Input: part model. Units: mm. Frame: model coordinates. Face numbers are marked on the shaded views. Give positions to 0.01 mm unless a question says otherwise; leave off trailing zeros. Write each loop counter-clockwise with the first axis right and the second up, starting at its lowest first coordinate (ties: lowest second). Pieces come first, ordered by that corner, then holes.
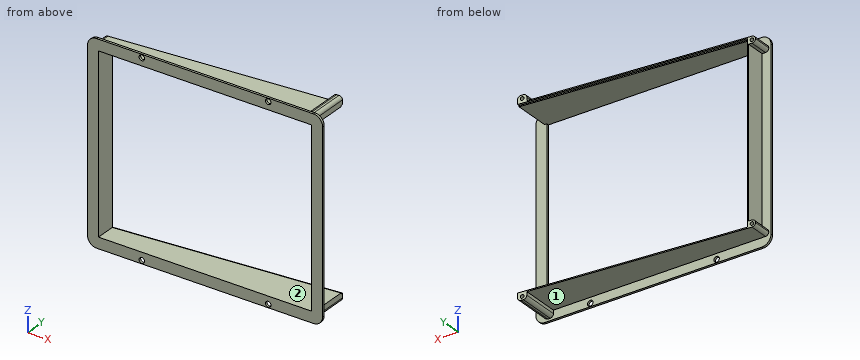
Autodesk Inventor part; units mm, degrees
ref_plane "YZ Plane" through (0, 0, 0) normal (1, 0, 0) x (0, 1, 0)
ref_plane "XZ Plane" through (0, 0, 0) normal (0, 1, 0) x (-1, 0, 0)
ref_plane "XY Plane" through (0, 0, 0) normal (0, 0, 1) x (1, 0, 0)
sketch "panelconnect" plane through (0, 0, 0) normal (0, 1, 0) x (-1, 0, 0)
  circle A0 centre (0, 0) radius 2.5
  circle A1 centre (115, 0) radius 2.5
  circle A2 centre (115, 173) radius 2.5
  circle A3 centre (0, 173) radius 2.5
  line L0 (57.2025, 240.8064) -> (94.1768, 240.8064)
  line L1 (94.1768, 240.8064) -> (82.9725, 250.4701)
  line L2 (82.9725, 250.4701) -> (82.9725, 230.5824)
  line L3 (82.9725, 230.5824) -> (94.1768, 240.8064)
  line L4 (172.5, 184) -> (-57.5, 184)
  line L5 (-57.5, 184) -> (-57.5, -11)
  line L6 (-57.5, -11) -> (172.5, -11)
  line L7 (172.5, -11) -> (172.5, 184)
  line L8 (-39.5, 166) -> (154.5, 166)
  line L9 (154.5, 166) -> (154.5, 7)
  line L10 (154.5, 7) -> (-39.5, 7)
  line L11 (-39.5, 7) -> (-39.5, 166)
  line L12 (164.5, 176) -> (-49.5, 176)
  line L13 (-49.5, 176) -> (-49.5, -3)
  line L14 (-49.5, -3) -> (164.5, -3)
  line L15 (164.5, -3) -> (164.5, 176)
  dimension "d0" = 5
  dimension "d1" = 5
  dimension "d3" = 5
  dimension "d7" = 5
  dimension "d11" = 195
  dimension "d14" = 18
  dimension "d15" = 10
  dimension "d54" = 115
  dimension "d55" = 57.5
  dimension "d56" = 57.5
  dimension "d57" = 230
  dimension "d58" = 173
  dimension "d61" = 11
  dimension "d62" = 57.5
  dimension "d64" = 57.5
  dimension "d65" = 11
extrude "panelExtrude" add sketch "panelconnect" along normal blind 2 contours L15 L14 L13 L12
sketch "Sketch2" plane through (0, 2, 0) normal (0, 1, 0) x (1, 0, 0)
  line L0 (39.5, -7) -> (39.5, -166)
  line L1 (-154.5, -166) -> (39.5, -166)
  line L2 (39.5, -166) -> (39.5, -7)
  line L3 (39.5, -7) -> (-154.5, -7)
  line L4 (-154.5, -7) -> (-154.5, -166)
  line L5 (41.5, -168) -> (-156.5, -168)
  line L6 (-156.5, -168) -> (-156.5, -5)
  line L7 (-156.5, -5) -> (41.5, -5)
  line L8 (41.5, -5) -> (41.5, -168)
  line L9 (39.5, -7) -> (64.2045, -7)
  line L10 (39.5, -166) -> (-154.5, -166)
  line L11 (39.5, -166) -> (69.5542, -166)
  line L12 (-156.5, -5) -> (-156.5, -168)
  line L13 (41.5, -168) -> (33.5, -168)
  line L14 (33.5, -168) -> (33.5, -174)
  line L15 (33.5, -174) -> (41.5, -174)
  line L16 (41.5, -174) -> (41.5, -168)
  line L17 (41.5, -5) -> (33.5, -5)
  line L18 (33.5, -5) -> (33.5, 1)
  line L19 (33.5, 1) -> (41.5, 1)
  line L20 (41.5, 1) -> (41.5, -5)
  circle A0 centre (37.5, -171) radius 1.55
  circle A1 centre (37.5, -2) radius 1.55
  line L21 (-156.5, -168) -> (-162.5, -168)
  line L22 (-162.5, -168) -> (-162.5, -162)
  line L23 (-162.5, -162) -> (-156.5, -162)
  line L24 (-156.5, -162) -> (-156.5, -168)
  line L25 (-156.5, -5) -> (-162.5, -5)
  line L26 (-162.5, -5) -> (-162.5, -11)
  line L27 (-162.5, -11) -> (-156.5, -11)
  line L28 (-156.5, -11) -> (-156.5, -5)
  circle A2 centre (-159.5, -165) radius 1.55
  circle A3 centre (-159.5, -8) radius 1.55
  point P0 (0, 0)
  point P1 (41.5, -166)
  point P2 (41.5, -7)
  point P3 (-156.5, -5)
  dimension "d18" = 2
  dimension "d28" = 8
  dimension "d29" = 6
  dimension "d30" = 6
  dimension "d34" = 3.1
  dimension "d35" = 3
  dimension "d36" = 4
  dimension "d37" = 3.1
  dimension "d38" = 3
  dimension "d39" = 4
  dimension "d42" = 6
  dimension "d43" = 6
  dimension "d44" = 6
  dimension "d45" = 6
  dimension "d46" = 3.1
  dimension "d47" = 3
  dimension "d48" = 3
  dimension "d49" = 3.1
  dimension "d50" = 3
  dimension "d51" = 3
extrude "bodyExtrude" add sketch "Sketch2" along normal blind 35 contours L3 L4 L1 L11 L8 L5 L6 L7 L9 | L7 L18 L19 L20 | L16 L15 L14 L5 | L6 L27 L26 L25 | L21 L22 L23 L6
sketch "Sketch3" plane through (-161.5, 2, 168) normal (0, 0, 1) x (1, 0, 0)
  line L0 (203, 0) -> (203, 35)
  line L1 (203, 35) -> (-34.1829, 14.2492)
  line L2 (203, 35) -> (441.0889, 35) construction
  line L3 (7, 35) -> (203, 35)
  line L4 (-1, 0) -> (-1, 35)
  line L5 (-1, 17.5) -> (-1, 35)
  line L6 (203, 35) -> (195, 35)
  line L7 (-1, 35) -> (203, 35)
  point P0 (161.5, -2)
  point P1 (-1, 17.1523)
  dimension "d22" = 175
extrude "baseAngle" cut sketch "Sketch3" against normal mid plane 398.4625
sketch "Sketch4" plane through (-161.5, 19.2398, 168) normal (-0.0872, 0.9962, 0) x (0.9962, 0.0872, 0)
  line L0 (7.0267, 161) -> (7.0267, 2)
  line L1 (7.0267, 2) -> (203.6093, 2)
  line L2 (203.6093, 2) -> (203.6093, 161)
  line L3 (203.6093, 161) -> (7.0267, 161)
  line L4 (7.0267, 161) -> (7.0267, 2)
  line L5 (6.0267, 162) -> (204.6093, 162)
  line L6 (204.6093, 162) -> (204.6093, 1)
  line L7 (204.6093, 1) -> (6.0267, 1)
  line L8 (6.0267, 1) -> (6.0267, 162)
  point P0 (159.2086, 168)
  point P1 (7.0267, 21.4312)
  dimension "d25" = 1
extrude "bodyDetent" cut sketch "Sketch4" against normal blind 2 contours L3 L2 L1 L0 | L5 L6 L7 L8
fillet "Fillet1" radius 8.35 4 edges at (49.5, 1, -3) (-164.5, 1, -3) (-164.5, 1, 176) (49.5, 1, 176)
fillet "Fillet2" radius 3 8 edges at (33.5, 19.15, 174) (41.5, 19.5, 174) (41.5, 19.5, -1) (33.5, 19.15, -1) (-162.5, 10.5762, 11) (-162.5, 10.5762, 5) (-162.5, 10.5762, 162) (-162.5, 10.5762, 168)
properties part number "mainBody"
Item 1: Section D-D (x = 0). Return loops of the section in (y, z), and give its area (3 significant figures).
Item 2: Section A-A (y = 8). Give the number of separate pieces and of enclosed holes in the cut face, and give its area (3 significant figures).
Item 3: Ray query, line 1 (Z direction, x = 37.5, y = 15); line 2 (Z direction, x = -43, y = 15); line 3 (Z direction, x = -115, y = 0.7). Return the intervals inside material, ascending.
Item 4: Mould query, pull axis Z, two halves, no side actions, for the marked faces 1 and 2. Classes: +Z half, -Z half, draft (parallel to the pull), parting line (faces both ways), or undercut.
Item 5: Section C-C (y = 28.5). Return loops of the section in (x, z).
Item 6: Pin query (flat end, axial travel): pin 1 (1.5 mm diameter, centred on x = 19, y = 33, fed in from -Z); pin 2 (8 mm diameter, centred on x = 0, z = 173, fed in from +Y); pin 3 (9.5 mm diameter, centred on x = -78.5, y = 27, fed in from +Z); pin 4 (4 mm diameter, centred on x = -93, y = 29, fed in from -Z). Return the tip coordinate at first contact, or that it passes through.
Item 7: Section B-B (z = 151). Return loops of the section in (x, y), and give its area (3 significant figures).
Solved:
1. outline: (0, -3) - (2, -3) - (2, -2.5) - (0, -2.5) - close; (0, 2.5) - (2, 2.5) - (2, 5) - (33.37, 5) - (33.37, 6) - (31.36, 6) - (31.36, 7) - (0, 7) - close; (0, 166) - (31.36, 166) - (31.36, 167) - (33.37, 167) - (33.37, 168) - (2, 168) - (2, 170.5) - (0, 170.5) - close; (0, 175.5) - (2, 175.5) - (2, 176) - (0, 176) - close
1. area: 141 mm2
2. separate pieces: 1
2. enclosed holes: 4
2. area: 1,230 mm2
3. line 1: z = -1 to 0.45, 3.55 to 7, 166 to 169.45, 172.55 to 174
3. line 2: z = 5 to 7, 166 to 168
3. line 3: z = -3 to -2.5, 2.5 to 7, 166 to 170.5, 175.5 to 176
4. face 1: -Z half
4. face 2: undercut
5. outline: (-55.66, 5) - (33.5, 5) - (33.5, 2) arc R3 ccw to (36.5, -1) - (38.5, -1) arc R3 ccw to (41.5, 2) - (41.5, 7) - (-32.69, 7) - (-32.69, 6) - (-55.66, 6) - close; (-55.66, 167) - (-32.69, 167) - (-32.69, 166) - (41.5, 166) - (41.5, 171) arc R3 ccw to (38.5, 174) - (36.5, 174) arc R3 ccw to (33.5, 171) - (33.5, 168) - (-55.66, 168) - close; hole circle Ø3.1 at (37.5, 2); hole circle Ø3.1 at (37.5, 171)
6. pin 1: stops at z = 5
6. pin 2: stops at y = 2
6. pin 3: stops at z = 168
6. pin 4: passes through
7. outline: (-164.5, 0) - (-154.5, 0) - (-154.5, 17.84) - (-155.32, 17.77) - (-155.5, 19.77) - (-156.5, 19.68) - (-156.5, 2) - (-164.5, 2) - close; (39.5, 0) - (49.5, 0) - (49.5, 2) - (39.5, 2) - close
7. area: 73.7 mm2
